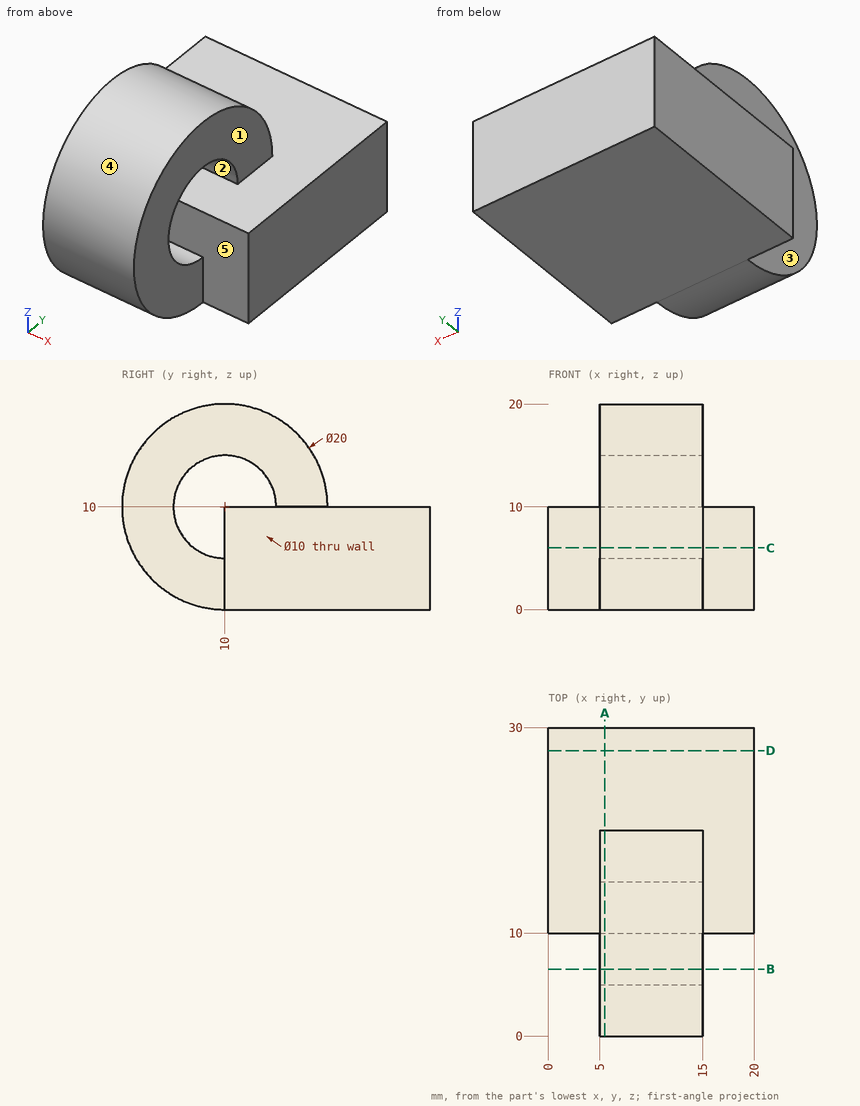
Geometry: see drawing. Coordinates: mm, zero at the bounding-box minimum. A direction names the side the tool comes from. Give positions to 0.01 mm unless a question says otherwise; leave off trailing zeros. Write each loop counter-clockwise with the first axis right and the second up, starting at its lowest first coordinate (ties: lowest second). Pieces come first, ordered by that corner, then holes. Notation, with made-up numbers: M -17.5,31.25 L 12.5,31.25 A20 cw 12.5,69.25 Z; hole C 54,6.25 d9. An arc over 180 degrees is marked long. Answer in a Markdown table with one row per item. Add a question column.
(1) First-contact query: pin 1 (5 mm diameter, centred on x = 16, z = 6.5, fed in from -Y); pin 2 (12 mm diameter, centred on x = 12, y = 20, fed in from -Z); pin 3 (4 mm diameter, centred on y = 17, z = 18, fed in from -X); pin 4 (4 mm diameter, centred on x = 7.5, y = 7, fed in from +Z). Flat tips, straight axial feed; report the tip coordinate or a pass-through.
(2) Section B-B on y = 6.5. Return loops of the section in (x, z), and give its area (3 significant figures).
(3) Reachability of the marked faces 1 and 2 from +Z, -Z, +X, -X, +Y, -Y: full face, straight path, thin tool, end or side. Return the list, or none.
(4) Mould query, pull axis Y, two halves, no side actions, for the marked faces 3, 4 and 5. Classes: +Y half, -Y half, draft (parallel to the pull), parting line (faces both ways), or undercut.
(5) Section D-D on y = 27.75. Return loops of the section in (x, z).
(6) Section A-A on x = 5.5. Return loops of the section in (y, z).
(7) Section C-C on z = 6. Return loops of the section in (x, y), and give its area (3 significant figures).
(8) Ray query, line 1 (Z direction, x = 2, y = 28.5); line 2 (X direction, y = 9.25, z = 16); line 3 (Z direction, x = 14, y = 7.25). Return the intervals inside material, ascending.
Result set:
| question | item | result |
|---|---|---|
| 1 | pin 1 | stops at y = 0.07 |
| 1 | pin 2 | stops at z = 0 |
| 1 | pin 3 | stops at x = 5 |
| 1 | pin 4 | stops at z = 19.95 |
| 2 | outline | M 5,0.63 L 15,0.63 L 15,6.43 L 5,6.43 Z; M 5,13.57 L 15,13.57 L 15,19.37 L 5,19.37 Z |
| 2 | area | 116 mm^2 |
| 3 | face 1 | +Z, +X, -Y |
| 3 | face 2 | +X, -X |
| 4 | face 3 | draft |
| 4 | face 4 | parting line |
| 4 | face 5 | undercut |
| 5 | outline | M 0,0 L 20,0 L 20,10 L 0,10 Z |
| 6 | outline | M 10,0 L 30,0 L 30,10 L 20,10 A10 ccw long Z; hole M 10,5 L 10,10 L 15,10 A5 ccw long Z |
| 7 | outline | M 0,10 L 20,10 L 20,30 L 0,30 Z; M 5,0.83 L 15,0.83 L 15,7 L 5,7 Z |
| 7 | area | 462 mm^2 |
| 8 | line 1 | z = 0 to 10 |
| 8 | line 2 | x = 5 to 15 |
| 8 | line 3 | z = 0.39 to 5.82, 14.18 to 19.61 |
